CAD build for the part. Positions are in the model's coordinates, mm. A direction names the side the tool comes from. Coordinates: 2 decimals unless noted, no trailing zeros. Order: outer loops, then holes, each group sorted by start corner. A loop starts at its lowest first (then second) coordinate and runs counter-clockwise, first axis right, second up. Notation, with made-up numbers: (39, 55) - (90, 55) arc R20 cw to (90, 71) - close; hole circle Ø3 at (73.25, -7). An arc over 180 degrees is marked (long way). Return JSON: item names as keys, results as strings.
Autodesk Inventor part; units mm, degrees
ref_plane "YZ Plane" through (0, 0, 0) normal (1, 0, 0) x (0, 1, 0)
ref_plane "XZ Plane" through (0, 0, 0) normal (0, 1, 0) x (-1, 0, 0)
ref_plane "XY Plane" through (0, 0, 0) normal (0, 0, 1) x (1, 0, 0)
sketch "Sketch1" plane through (0, 0, 0) normal (0, 0, 1) x (1, 0, 0)
  point P0 (0, 0)
sketch "Sketch2" plane through (0, 0, 0) normal (0, 0, 1) x (1, 0, 0)
  line L0 (94.9998, -95.0001) -> (-94.9998, -95.0001)
  line L1 (-94.9998, -95.0001) -> (-94.9998, 95.0001)
  line L2 (-94.9998, 95.0001) -> (94.9998, 95.0001)
  line L3 (94.9998, 95.0001) -> (94.9998, -95.0001)
  line L4 (94.9998, -95.0001) -> (-94.9998, 95.0001) construction
  line L5 (-94.9998, -95.0001) -> (94.9998, 95.0001) construction
  point P0 (0, 0)
extrude "Extrusion1" add sketch "Sketch2" along normal blind 3
sketch "Sketch3" plane through (0, 0, 3) normal (0, 0, 1) x (1, 0, 0)
  circle A0 centre (70, 80) radius 1.5001
  circle A1 centre (70, -80) radius 1.5001
  circle A2 centre (-70, 80) radius 1.5001
  circle A3 centre (-70, -80) radius 1.5001
extrude "Extrusion2" cut sketch "Sketch3" against normal blind 3
fillet "Fillet1" radius 25 1 edges at (94.9998, 95.0001, 1.5)
fillet "Fillet2" radius 25 1 edges at (94.9998, -95.0001, 1.5)
fillet "Fillet3" radius 25 1 edges at (-94.9998, -95.0001, 1.5)
fillet "Fillet4" radius 25 1 edges at (-94.9998, 95.0001, 1.5)
sketch "Pi mount holes" plane through (0, 0, 3) normal (0, 0, 1) x (1, 0, 0)
  circle A0 centre (24, -30.5) radius 1.2502
  circle A1 centre (-34, -30.5) radius 1.2502
  circle A2 centre (-34, -79.5) radius 1.2502
  circle A3 centre (24, -79.5) radius 1.2502
sketch "B205 mount holes" plane through (0, 0, 3) normal (0, 0, 1) x (1, 0, 0)
  circle A0 centre (20.32, 30.48) radius 1.5002
  circle A1 centre (-45.72, 30.48) radius 1.5002
  circle A2 centre (-45.72, -12.7) radius 1.5002
  circle A3 centre (20.32, -12.7) radius 1.5002
sketch "RM3100 mount holes" plane through (0, 0, 3) normal (0, 0, 1) x (1, 0, 0)
  circle A0 centre (0, 9) radius 0.9999
  circle A1 centre (0, -9) radius 0.9999
sketch "Pololu mount holes" plane through (0, 0, 3) normal (0, 0, 1) x (1, 0, 0)
  circle A0 centre (59.5, 87.75) radius 1.2501
  circle A1 centre (44.5, 87.75) radius 1.2501
  circle A2 centre (44.5, 52.25) radius 1.2501
  circle A3 centre (59.5, 52.25) radius 1.2501
  circle A4 centre (-42.5, -52.25) radius 1.2501
  circle A5 centre (-57.5, -52.25) radius 1.2501
  circle A6 centre (-57.5, -87.75) radius 1.2501
  circle A7 centre (-42.5, -87.75) radius 1.2501
sketch "B205 cable cutout" plane through (0, 0, 3) normal (0, 0, 1) x (1, 0, 0)
  line L0 (-76.0426, -14.5593) -> (-76.0426, 37.4411) construction
  line L1 (-81.5424, -9.0595) -> (-81.5424, 31.9413)
  line L2 (-70.5428, 31.9413) -> (-70.5428, -9.0595)
  arc A0 (-81.5424, -9.0595) -> (-70.5428, -9.0595) centre (-76.0426, -9.0595) ccw
  arc A1 (-70.5428, 31.9413) -> (-81.5424, 31.9413) centre (-76.0426, 31.9413) ccw
  point P0 (0, 0)
  point P1 (-76.0426, 11.4409)
sketch "Pi cable cutout" plane through (0, 0, 3) normal (0, 0, 1) x (1, 0, 0)
  line L0 (65.7382, -60.7056) -> (65.7382, 5.2939) construction
  line L1 (60.7378, -55.7052) -> (60.7378, 0.2935)
  line L2 (70.7387, 0.2935) -> (70.7387, -55.7052)
  arc A0 (60.7378, -55.7052) -> (70.7387, -55.7052) centre (65.7382, -55.7052) ccw
  arc A1 (70.7387, 0.2935) -> (60.7378, 0.2935) centre (65.7382, 0.2935) ccw
  point P0 (0, 0)
  point P1 (65.7382, -27.7058)
sketch "Imperial standoffs" plane through (0, 0, 3) normal (0, 0, 1) x (1, 0, 0)
  circle A0 centre (80, 80) radius 1.4302
  circle A1 centre (-80, -80) radius 1.4302
  circle A2 centre (80, -80) radius 1.4302
  circle A3 centre (-80, 80) radius 1.4302
extrude "Bottom payload mount holes" cut sketch "Imperial standoffs" against normal blind 10
sketch "FC mount" plane through (0, 0, 3) normal (0, 0, 1) x (1, 0, 0)
  circle A0 centre (-22.5, 22.5) radius 1.4999
  circle A1 centre (-22.5, -22.5) radius 1.4999
  circle A2 centre (22.5, -22.5) radius 1.4999
  circle A3 centre (22.5, 22.5) radius 1.4999
  circle A4 centre (-10.75, 13.75) radius 1.2498
  circle A5 centre (-10.75, -7.75) radius 1.2498
  circle A6 centre (10.75, -7.75) radius 1.2498
  circle A7 centre (10.75, 13.75) radius 1.2498
  point P0 (0, 0)
sketch "FC cable cutouts" plane through (0, 0, 3) normal (0, 0, 1) x (1, 0, 0)
  line L0 (-65, -20.0003) -> (-65, 20.0003) construction
  line L1 (-58.4981, -20.0003) -> (-58.4981, 20.0003)
  line L2 (-71.5019, 20.0003) -> (-71.5019, -20.0003)
  arc A0 (-71.5019, -20.0003) -> (-58.4981, -20.0003) centre (-65, -20.0003) ccw
  arc A1 (-58.4981, 20.0003) -> (-71.5019, 20.0003) centre (-65, 20.0003) ccw
  line L3 (65, -20.0003) -> (65, 20.0003) construction
  line L4 (71.5019, -20.0003) -> (71.5019, 20.0003)
  line L5 (58.4981, 20.0003) -> (58.4981, -20.0003)
  arc A2 (58.4981, -20.0003) -> (71.5019, -20.0003) centre (65, -20.0003) ccw
  arc A3 (71.5019, 20.0003) -> (58.4981, 20.0003) centre (65, 20.0003) ccw
  arc A4 (-20.0003, 76.5019) -> (-20.0003, 63.4981) centre (-20.0003, 70) ccw
  line L6 (-20.0003, 63.4981) -> (20.0003, 63.4981)
  line L7 (20.0003, 70) -> (-20.0003, 70) construction
  line L8 (20.0003, 76.5019) -> (-20.0003, 76.5019)
  arc A5 (20.0003, 63.4981) -> (20.0003, 76.5019) centre (20.0003, 70) ccw
  line L9 (20.0003, -63.4981) -> (-20.0003, -63.4981)
  line L10 (20.0003, -70) -> (-20.0003, -70) construction
  line L11 (-20.0003, -76.5019) -> (20.0003, -76.5019)
  arc A6 (20.0003, -76.5019) -> (20.0003, -63.4981) centre (20.0003, -70) ccw
  arc A7 (-20.0003, -63.4981) -> (-20.0003, -76.5019) centre (-20.0003, -70) ccw
  point P0 (0, 0)
sketch "Skid cutouts" plane through (0, 0, 3) normal (0, 0, 1) x (1, 0, 0)
  line L0 (75, 0) -> (75, 39.9996)
  line L1 (75, 39.9996) -> (75, 0)
  line L2 (75, 0) -> (75, -40)
  line L3 (94.9998, -70.0001) -> (94.9998, 70.0001)
  arc A0 (94.9998, 70.0001) -> (75, 39.9996) centre (106.9986, 40.3344) ccw
  arc A1 (69.9998, -95.0001) -> (94.9998, -70.0001) centre (69.9998, -70.0001) ccw
  arc A2 (75, -40) -> (94.9998, -70.0001) centre (106.9987, -40.3344) ccw
  line L4 (-75, 0) -> (-75, -39.9996)
  line L5 (-75, -39.9996) -> (-75, 0)
  line L6 (-75, 0) -> (-75, 40)
  arc A3 (-94.9998, -70.0001) -> (-75, -39.9996) centre (-106.9986, -40.3344) ccw
  arc A4 (-75, 40) -> (-94.9998, 70.0001) centre (-106.9987, 40.3344) ccw
  line L7 (-94.9998, 70.0001) -> (-94.9998, -70.0001)
  line L8 (-94.9998, -70.0001) -> (-94.9998, 70.0001)
  line L9 (-94.9998, 70.0001) -> (-94.9998, -70.0001)
  point P0 (0, 0)
extrude "Extrusion10" cut sketch "Skid cutouts" against normal blind 10
extrude "Extrusion11" cut sketch "FC cable cutouts" against normal blind 10
extrude "Extrusion12" cut sketch "Pololu mount holes" against normal blind 10
extrude "Extrusion13" cut sketch "FC mount" against normal blind 10
properties part number "payload_bay_square_FC" material "ABS Plastic"
Item 1: Band-saw the part on D-D, the plane z = 0.95. Count the separate pieces of the cut face and the enclosed holes in it, then the cut area to 3 significant figures.
Findings below:
{"separate pieces": "1", "enclosed holes": "28", "area": "27,900 mm²"}
Item 2: Drop flat-ended pins along their axis: P1, Ø2.5, axis at x = 80, y = 80, coming from the -Z side; P2, Ø3, axis at x = 59.5, y = 52.25, coming from the -Z side. Give the stop position or say it passes through.
Findings below:
{"P1": "passes through", "P2": "stops at z = 0"}
Item 3: Band-saw the part on B-B, the plane x = -65. List the corners of the cut face in (y, z), then the cut area to 3 significant figures.
Findings below:
{"outline": "(-95, 0) - (-26.5, 0) - (-26.5, 3) - (-95, 3) - close; (26.5, 0) - (95, 0) - (95, 3) - (26.5, 3) - close", "area": "411 mm²"}
Item 4: Mould opens along X. For faces 4 (the cylindrical face through (26.5, -70.1, 1.5)), 5 (the cylindrical face through (-87.871, -87.482, 1.521)), 6 (the flat face through (-1, 1, 0)), 7 (the cylindrical face through (-26.5, 70.1, 1.5)) say: released by +X, released by -X, zero draft, split by the parting line, or undercut.
Findings below:
{"face 4": "undercut", "face 5": "released by -X", "face 6": "zero draft", "face 7": "undercut"}
Item 5: Wall check: L1, parallel to Y at x = -10.75, z = 2.2; L2, parallel to Y at x = -15, z = 1.65; L3, parallel to Y at x = -57.5, z = 2.3. Give the ranges that are in metal, low to high. Write a range as [from, to].
Findings below:
{"L1": "y = [-95, -76.5], [-63.5, -9], [-6.5, 12.5], [15, 63.5], [76.5, 95]", "L2": "y = [-95, -76.5], [-63.5, 63.5], [76.5, 95]", "L3": "y = [-95, -89], [-86.5, -53.5], [-51, 95]"}
Item 6: Band-saw the part on C-C, the plane y = -72.5. List the corners of the cut face in (x, z).
Findings below:
{"outline": "(-94.87, 0) - (-26, 0) - (-26, 3) - (-94.87, 3) - close; (26, 0) - (94.87, 0) - (94.87, 3) - (26, 3) - close"}
Item 7: Band-saw the part on A-A, the plane x = -5. List the corners of the cut face in (y, z).
Findings below:
{"outline": "(-95, 0) - (-76.5, 0) - (-76.5, 3) - (-95, 3) - close; (-63.5, 0) - (63.5, 0) - (63.5, 3) - (-63.5, 3) - close; (76.5, 0) - (95, 0) - (95, 3) - (76.5, 3) - close"}
Item 8: Which spindle directions (+Z, -Z, +X, -X, +Y, -Y) get a long thin tool onto all of the face, cutting with end or side? Do faces 1 (the cylindrical face through (80.225, -57.861, 1.521)), 2 (the cylindrical face through (-26.5, -69.9, 1.5)), 3 (the cylindrical face through (-80.225, 57.861, 1.521)). Say none if no direction does.
Findings below:
{"face 1": "+Z, -Z, +X", "face 2": "+Z, -Z", "face 3": "+Z, -Z, -X"}
